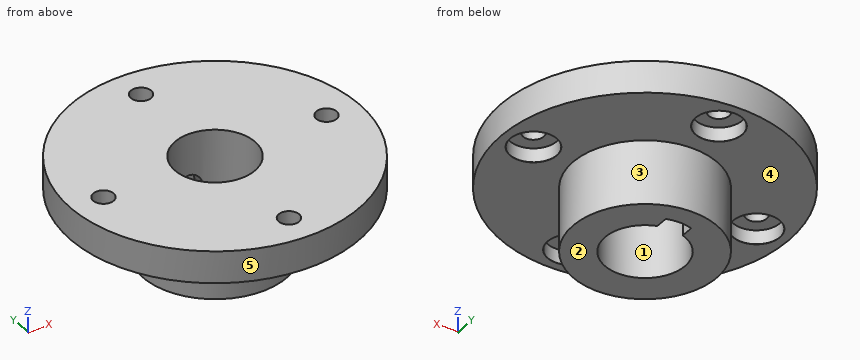
from build123d import *

# Parameters (mm, degrees)
SKETCH1_R                              = 22.5
SKETCH1_R_2                            = 12.5
BOSS_EXTRUDE1_DEPTH                    = 20
BOSS_EXTRUDE2_START                    = 10
SKETCH2_R                              = 45
SKETCH2_R_2                            = 12.5
BOSS_EXTRUDE2_DEPTH                    = 10
CUT_EXTRUDE1_START                     = 11
CUT_EXTRUDE1_DEPTH                     = 4.842719182
CUT_EXTRUDE1_START_2                   = -21
CUT_EXTRUDE1_2_DEPTH                   = 18.000002419
CUT_EXTRUDE1_START_3                   = 15.842719282
CUT_EXTRUDE1_3_DEPTH                   = 1.157280718
CBORE_FOR_M6_HEX_HEAD_BOLT1_AT_2_COUNT = 2
CBORE_FOR_M6_HEX_HEAD_BOLT1_AT_2_PITCH = 49.497474683
CBORE_FOR_M6_HEX_HEAD_BOLT1_AT_3_COUNT = 2
CBORE_FOR_M6_HEX_HEAD_BOLT1_AT_3_PITCH = 70
CBORE_FOR_M6_HEX_HEAD_BOLT1_AT_4_COUNT = 2
CBORE_FOR_M6_HEX_HEAD_BOLT1_AT_4_PITCH = 49.497474683


with BuildPart() as part:
    # Sketch1 → Boss-Extrude1 (new body)
    with BuildSketch(Plane.XY):
        Circle(SKETCH1_R)
        Circle(SKETCH1_R_2, mode=Mode.SUBTRACT)
    extrude(amount=-BOSS_EXTRUDE1_DEPTH)

    # Sketch2 → Boss-Extrude2 (add)
    with BuildSketch(Plane.XY.offset(BOSS_EXTRUDE2_START)):
        Circle(SKETCH2_R)
        Circle(SKETCH2_R_2, mode=Mode.SUBTRACT)
    extrude(amount=-BOSS_EXTRUDE2_DEPTH)

    # Cut-Extrude1: read off the stored shape, not the designer's step
    # Cut-Extrude1 outline → Cut-Extrude1 (cut)
    with BuildSketch(Plane(origin=(0, 0, 0), x_dir=(1, 0, 0), z_dir=(0, 1, 0)).offset(CUT_EXTRUDE1_START)):
        with BuildLine():
            add(Edge.make_bspline(
                [(4, 7), (4.000000645, 5.935618893), (3.56110042, 4.904383726), (2.096294231, 3.439297629), (1.055347946, 3.001083541), (-1.047099738, 2.998915861), (-2.090363581, 3.433909578), (-3.564946099, 4.907687175), (-4, 5.935522054), (-4, 6.999997575)],
                knots=[0, 0, 0, 0, 0.25, 0.25, 0.5, 0.5, 0.75, 0.75, 1, 1, 1, 1], degree=3))
            Line((4, 7), (4, 20))
            Line((4, 20), (-4, 20))
            Line((-4, 20), (-4, 6.999997575))
        make_face()
    extrude(amount=CUT_EXTRUDE1_DEPTH, mode=Mode.SUBTRACT)

    # Cut-Extrude1 2 outline → Cut-Extrude1 2 (cut)
    with BuildSketch(Plane.XY.offset(CUT_EXTRUDE1_START_2)):
        with BuildLine():
            Line((-4, 15.842719282), (4, 15.842719282))
            ThreePointArc((4, 15.842719282), (0, 16.5), (-4, 15.842719282))
        make_face()
    extrude(amount=CUT_EXTRUDE1_2_DEPTH, mode=Mode.SUBTRACT)

    # Cut-Extrude1 3 outline → Cut-Extrude1 3 (add)
    with BuildSketch(Plane(origin=(0, 0, 0), x_dir=(1, 0, 0), z_dir=(0, 1, 0)).offset(CUT_EXTRUDE1_START_3)):
        with BuildLine():
            Line((-4, 2.999997581), (0.000204294, 2.999997681))
            add(Edge.make_bspline(
                [(0.000204294, 2.999997681), (-1.049692709, 2.999997676), (-2.091279995, 3.434825492), (-3.564946099, 4.907687175), (-4, 5.935522054), (-4, 6.999997575)],
                knots=[0.500310737, 0.500310737, 0.500310737, 0.500310737, 0.75, 0.75, 1, 1, 1, 1], degree=3))
            Line((-4, 6.999997575), (-4, 2.999997581))
        make_face()
        with BuildLine():
            add(Edge.make_bspline(
                [(4, 7), (4.000000645, 5.935618893), (3.56110042, 4.904383726), (2.096294231, 3.439297629), (1.055347946, 3.001083541), (0.002817488, 2.999998354), (0.001510885, 2.999997681), (0.000204294, 2.999997681)],
                knots=[0, 0, 0, 0, 0.25, 0.25, 0.5, 0.5, 0.500310737, 0.500310737, 0.500310737, 0.500310737], degree=3))
            Line((0.000204294, 2.999997681), (4, 2.999997581))
            Line((4, 2.999997581), (4, 7))
        make_face()
    extrude(amount=CUT_EXTRUDE1_3_DEPTH)

    # Sketch5 → CBORE for M6 Hex Head Bolt1 (revolve, cut)
    with BuildSketch(Plane.YZ.offset(35)):
        Polygon((0, 0), (0, 10), (3.2, 10), (3.2, 4.38), (7.275, 4.38), (7.275, 0.025), (7.3, 0), align=None)
    cbore_for_m6_hex_head_bolt1 = revolve(axis=Axis((35, 0, -6.35), (0, 0, 1)), mode=Mode.SUBTRACT)

    # CBORE for M6 Hex Head Bolt1 at 2: CBORE for M6 Hex Head Bolt1 ×2
    with Locations(*[Vector(-0.7071067811865277, 0.7071067811865673, 0) * (i * CBORE_FOR_M6_HEX_HEAD_BOLT1_AT_2_PITCH) for i in range(1, CBORE_FOR_M6_HEX_HEAD_BOLT1_AT_2_COUNT)]):
        add(cbore_for_m6_hex_head_bolt1, mode=Mode.SUBTRACT)

    # CBORE for M6 Hex Head Bolt1 at 3: CBORE for M6 Hex Head Bolt1 ×2
    with Locations(*[(-i * CBORE_FOR_M6_HEX_HEAD_BOLT1_AT_3_PITCH, 0, 0) for i in range(1, CBORE_FOR_M6_HEX_HEAD_BOLT1_AT_3_COUNT)]):
        add(cbore_for_m6_hex_head_bolt1, mode=Mode.SUBTRACT)

    # CBORE for M6 Hex Head Bolt1 at 4: CBORE for M6 Hex Head Bolt1 ×2
    with Locations(*[Vector(-0.7071067811865674, -0.7071067811865276, 0) * (i * CBORE_FOR_M6_HEX_HEAD_BOLT1_AT_4_PITCH) for i in range(1, CBORE_FOR_M6_HEX_HEAD_BOLT1_AT_4_COUNT)]):
        add(cbore_for_m6_hex_head_bolt1, mode=Mode.SUBTRACT)


solid = part.part
For this review, take the finished solid that the model builds, in its own axes (mm). Face numbers are marked on the shaded views. A direction names the side the tool comes from. Coordinates: 2 decimals unless noted, no trailing zeros. Loops run counter-clockwise (first coordinate to the right, second up) from the corner with the lowest first, then second, coordinate; pieces in that order, holes last. Notation, with made-up numbers: (23, -14.75) - (46, -14.75) arc R30 cw to (46, 19.25) - close; hole circle Ø3 at (88.25, 28). An arc over 180 degrees is marked (long way). Use a Markdown table: item, result. Add a question column.
Item 1: We need section B-B (y = -35). Give the boundary of the cut face in (x, z) (3 decimals).
Item 2: Tool access review of the marked faces 4 and 5: name each direction out of +Z, -Z, +X, -X, +Y, -Y from which nothing blocks a thin tool from reaching the whole face with its end or side.
Item 3: We need section C-C (z = -16). Give the boundary of the cut face in (x, y), and give its area (3 significant figures).
Item 4: Mouldability with a two-part tool opening along X and no side actions: class the marked faces 1, 2 and 3 as pulls with the +X half, pulls with the -X half, needs draft (parallel to the pull), parting line crosses it, or undercut.
Item 5: We need section A-A (y = 0). Give the number of separate pieces and of enclosed holes in the cut face, and give its area (3 significant figures).
Item 6: For line 1 (X direction, y = 2.5, z = 1); line 2 (Z direction, x = 9.5, y = 27.5); line 3 (X direction, y = -8.5, z = 8.5), list the stretches that pass through material, from the lowest coordinate up.
Item 7: Insertion check: pin 1 Ø11.5 at (x, y) = (-3, -35.5) entering from -Z; pin 2 Ø1.2 at (y, z) = (13.5, -11.5) entering from +X; pin 3 Ø1.5 at (y, z) = (-13, -9.5) entering from +X; pin 4 Ø8.5 at (x, y) = (0, 35) entering from +Z. Each pin has a flat end and moves straight along its axis. Give the tip position at first contact, or say it passes through.
Results list:
| question | item | result |
|---|---|---|
| 1 | outline | (-28.284, 0) - (-7.3, 0) - (-7.275, 0.025) - (-7.275, 4.38) - (-3.2, 4.38) - (-3.2, 10) - (-28.284, 10) - close; (3.2, 4.38) - (7.275, 4.38) - (7.275, 0.025) - (7.3, 0) - (28.284, 0) - (28.284, 10) - (3.2, 10) - close |
| 2 | face 4 | -Z |
| 2 | face 5 | +Z, -Z |
| 3 | outline | circle Ø45 at (0, 0); hole (-4, 11.84) arc R12.5 ccw (long way) to (4, 11.84) - (4, 15.84) arc R12.5 ccw to (-4, 15.84) - close |
| 3 | area | 1,070 mm^2 |
| 4 | face 1 | undercut |
| 4 | face 2 | needs draft |
| 4 | face 3 | parting line crosses it |
| 5 | separate pieces | 4 |
| 5 | enclosed holes | 0 |
| 5 | area | 851 mm^2 |
| 6 | line 1 | x = -44.93 to -41.83, -28.17 to -12.25, 12.25 to 28.17, 41.83 to 44.93 |
| 6 | line 2 | z = 0 to 10 |
| 6 | line 3 | x = -44.19 to -9.17, 9.17 to 44.19 |
| 7 | pin 1 | stops at z = 0 |
| 7 | pin 2 | stops at x = 18.43 |
| 7 | pin 3 | stops at x = 18.87 |
| 7 | pin 4 | stops at z = 10 |
